from build123d import *

# Parameters (mm, degrees)
SKETCH1_W           = 25
SKETCH1_H           = 125
SKETCH1_W_2         = 450
SKETCH1_H_2         = 25
SKETCH1_R           = 3.5
BOSS_EXTRUDE1_DEPTH = 6.35
SKETCH2_W           = 140.00000048
SKETCH2_H           = 465.00000048
CUT_EXTRUDE1_DEPTH  = 514.909352415
SKETCH3_W           = 3.25
SKETCH3_H           = 500
CUT_EXTRUDE2_DEPTH  = 514.909352415
FILLET1_R           = 2.13
FILLET2_R           = 5


with BuildPart() as part:
    # Sketch1 → Boss-Extrude1 (new body)
    # profile 1 of 6: a face of its own
    with BuildSketch(Plane(origin=(0, 0, 0), x_dir=(0, 1, 0), z_dir=(0, 0, 1))):
        Polygon((-12.5, 137.5), (12.5, 137.5), (462.5, 137.5), (487.5, 137.5), (487.5, 162.5), (-12.5, 162.5), align=None)
    # profile 2 of 6: a face of its own
    with BuildSketch(Plane(origin=(0, 0, 0), x_dir=(0, 1, 0), z_dir=(0, 0, 1))):
        with Locations((0, 75)):
            Rectangle(SKETCH1_W, SKETCH1_H)
    # profile 3 of 6: a face of its own
    with BuildSketch(Plane(origin=(0, 0, 0), x_dir=(0, 1, 0), z_dir=(0, 0, 1))):
        with Locations((237.5, 0)):
            Rectangle(SKETCH1_W_2, SKETCH1_H_2)
    # profile 4 of 6: a face of its own
    with BuildSketch(Plane(origin=(0, 0, 0), x_dir=(0, 1, 0), z_dir=(0, 0, 1))):
        with Locations((475, 75)):
            Rectangle(SKETCH1_W, SKETCH1_H)
    # profile 5 of 6: a face of its own
    with BuildSketch(Plane(origin=(0, 0, 0), x_dir=(0, 1, 0), z_dir=(0, 0, 1))):
        with Locations((475, 0)):
            Rectangle(SKETCH1_W, SKETCH1_H_2)
        with Locations(Location((475, 0, 0), (0, 0, 270))):
            Circle(SKETCH1_R, mode=Mode.SUBTRACT)
    # profile 6 of 6: a face of its own
    with BuildSketch(Plane(origin=(0, 0, 0), x_dir=(0, 1, 0), z_dir=(0, 0, 1))):
        Rectangle(SKETCH1_W, SKETCH1_H_2)
        with Locations(Location((0, 0, 0), (0, 0, 270))):
            Circle(SKETCH1_R, mode=Mode.SUBTRACT)
    extrude(amount=BOSS_EXTRUDE1_DEPTH)

    # Sketch2 → Cut-Extrude1 (cut, through all)
    with BuildSketch(Plane.XY.offset(6.35)):
        with Locations((-75, 237.5)):
            Rectangle(SKETCH2_W, SKETCH2_H)
    extrude(amount=-CUT_EXTRUDE1_DEPTH, mode=Mode.SUBTRACT)

    # Sketch3 → Cut-Extrude2 (cut, through all)
    with BuildSketch(Plane.XY.offset(6.35)):
        with Locations((-160.875, 237.5)):
            Rectangle(SKETCH3_W, SKETCH3_H)
    extrude(amount=-CUT_EXTRUDE2_DEPTH, mode=Mode.SUBTRACT)

    # Fillet1
    fillet1_edges = [part.edges().sort_by_distance(p)[0] for p in [
        (12.5, 487.5, 3.175),
        (12.5, -12.5, 3.175),
        (-159.25, 487.5, 3.175),
        (-159.25, -12.5, 3.175),
    ]]
    fillet(fillet1_edges, radius=FILLET1_R)

    # Fillet2
    fillet2_edges = [part.edges().sort_by_distance(p)[0] for p in [
        (-4.99999976, 470.00000024, 3.175),
        (-4.99999976, 4.99999976, 3.175),
        (-145.00000024, 4.99999976, 3.175),
        (-145.00000024, 470.00000024, 3.175),
    ]]
    fillet(fillet2_edges, radius=FILLET2_R)


solid = part.part
The listing builds one solid part. Answer for the finished solid, in the listing's coordinates (mm). Round coordinates to 2 decimals unless told otherwise and drop trailing zeros. Order: outer loops, then holes, each group sorted by start corner. A loop starts at its lowest first (then second) coordinate and runs counter-clockwise, first axis right, second up. Notation, with made-up numbers: (-4.5, 83) - (54.5, 83) arc R16 cw to (54.5, 105) - close; hole circle Ø8 at (-1.75, 44). An arc over 180 degrees is marked (long way). Write item = value, one per line. Start each with the question number.
1) Section C-C, the plane z = 5 is taken. Write down the section's boundary in (x, y), plus the area to 3 significant figures.
2) Given pin 1 (5.5 mm diameter, centred on x = 0, y = 0, fed in from +Z); pin 2 (9 mm diameter, centred on x = 0, y = 475, fed in from +Z), each flat-ended and moving along its own axis, determine where each tip first touches the part or whether it passes through.
3) Straight lines are drawn through the part: L1, parallel to Y at x = 0, z = 2; L2, parallel to Y at x = -17.5, z = 1.5; L3, parallel to X at y = 196.5, z = 3.75. For each, find the intervals that lie inside material, in ascending order.
4) Section A-A, the plane y = 353 is taken. Write down the section's boundary in (x, z), plus the area to 3 significant figures.
5) Section B-B, the plane x = -65.5 is taken. Write down the section's boundary in (y, z).
Results list:
q1.outline = (-159.25, -10.37) arc R2.13 ccw to (-157.12, -12.5) - (10.37, -12.5) arc R2.13 ccw to (12.5, -10.37) - (12.5, 485.37) arc R2.13 ccw to (10.37, 487.5) - (-157.12, 487.5) arc R2.13 ccw to (-159.25, 485.37) - close; hole (-145, 10) arc R5 ccw to (-140, 5) - (-10, 5) arc R5 ccw to (-5, 10) - (-5, 465) arc R5 ccw to (-10, 470) - (-140, 470) arc R5 ccw to (-145, 465) - close; hole circle Ø7 at (0, 0); hole circle Ø7 at (0, 475)
q1.area = 20,700 mm^2
q2.pin_1 = through
q2.pin_2 = 6.35
q3.L1 = -12.5 to -3.5, 3.5 to 471.5, 478.5 to 487.5
q3.L2 = -12.5 to 5, 470 to 487.5
q3.L3 = -159.25 to -145, -5 to 12.5
q4.outline = (-159.25, 0) - (-145, 0) - (-145, 6.35) - (-159.25, 6.35) - close; (-5, 0) - (12.5, 0) - (12.5, 6.35) - (-5, 6.35) - close
q4.area = 202 mm^2
q5.outline = (-12.5, 0) - (5, 0) - (5, 6.35) - (-12.5, 6.35) - close; (470, 0) - (487.5, 0) - (487.5, 6.35) - (470, 6.35) - close
